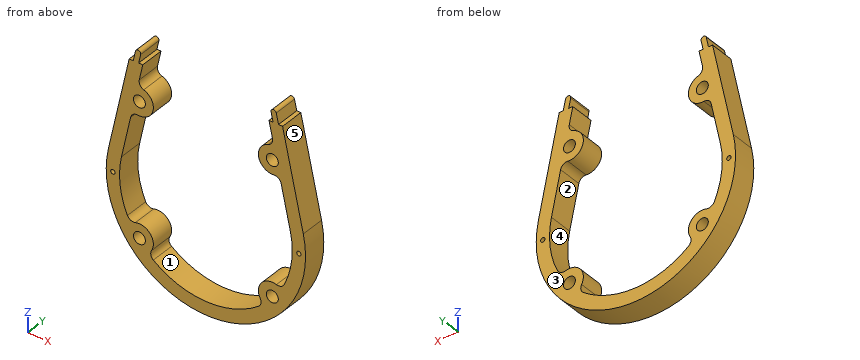
from build123d import *

# Parameters (mm, degrees)
SKETCH1_R           = 4.5
SKETCH1_R_2         = 1.65
BOSS_EXTRUDE1_DEPTH = 18


with BuildPart() as part:
    # Sketch1 → Boss-Extrude1 (new body)
    with BuildSketch(Plane(origin=(0, 0, 0), x_dir=(1, 0, 0), z_dir=(0, 1, 0))):
        with BuildLine():
            Line((-57.71713569, -88), (-54.647909803, -88))
            Line((-54.647909803, -88), (-52.972729242, -95.753217476))
            ThreePointArc((-52.972729242, -95.753217476), (-50.595460167, -97.285729058), (-49.062948585, -94.908459984))
            Line((-49.062948585, -94.908459984), (-50.555608621, -88))
            Line((-50.555608621, -88), (-47.486382735, -88))
            Line((-47.486382735, -88), (-50.121259231, -75.805033701))
            ThreePointArc((-50.121259231, -75.805033701), (-49.566331597, -72.252851185), (-46.771441988, -69.991316888))
            ThreePointArc((-46.771441988, -69.991316888), (-39.736825778, -57.782511582), (-51.184371295, -49.567010753))
            ThreePointArc((-51.184371295, -49.567010753), (-54.663630533, -48.661085559), (-56.635583446, -45.654867501))
            Line((-56.635583446, -45.654867501), (-63.533935661, -13.727309256))
            ThreePointArc((-63.533935661, -13.727309256), (-64.607519764, 7.132207931), (-59.0097537, 27.255255792))
            ThreePointArc((-59.0097537, 27.255255792), (-56.52196193, 29.718486659), (-53.028431594, 29.94621454))
            ThreePointArc((-53.028431594, 29.94621454), (-41.800877501, 33.440702001), (-40.856206486, 45.161495924))
            ThreePointArc((-40.856206486, 45.161495924), (-41.400905456, 48.61980725), (-39.543854024, 51.587630387))
            ThreePointArc((-39.543854024, 51.587630387), (0, 65), (39.543854024, 51.587630387))
            ThreePointArc((39.543854024, 51.587630387), (41.400905456, 48.61980725), (40.856206486, 45.161495924))
            ThreePointArc((40.856206486, 45.161495924), (41.800877501, 33.440702001), (53.028431594, 29.94621454))
            ThreePointArc((53.028431594, 29.94621454), (56.52196193, 29.718486659), (59.0097537, 27.255255792))
            ThreePointArc((59.0097537, 27.255255792), (64.607519764, 7.132207931), (63.533935661, -13.727309256))
            Line((63.533935661, -13.727309256), (56.635583446, -45.654867501))
            ThreePointArc((56.635583446, -45.654867501), (54.663630533, -48.661085559), (51.184371295, -49.567010753))
            ThreePointArc((51.184371295, -49.567010753), (39.736825778, -57.782511582), (46.771441988, -69.991316888))
            ThreePointArc((46.771441988, -69.991316888), (49.566331597, -72.252851185), (50.121259231, -75.805033701))
            Line((50.121259231, -75.805033701), (47.486382735, -88))
            Line((47.486382735, -88), (50.555608621, -88))
            Line((50.555608621, -88), (49.062948585, -94.908459984))
            ThreePointArc((49.062948585, -94.908459984), (50.595460167, -97.285729058), (52.972729242, -95.753217476))
            Line((52.972729242, -95.753217476), (54.647909803, -88))
            Line((54.647909803, -88), (57.71713569, -88))
            Line((57.71713569, -88), (73.308387301, -15.839202988))
            ThreePointArc((73.308387301, -15.839202988), (0, 75), (-73.308387301, -15.839202988))
            Line((-73.308387301, -15.839202988), (-57.71713569, -88))
        make_face()
        with Locations((-50, -60)):
            Circle(SKETCH1_R, mode=Mode.SUBTRACT)
        with Locations((50, -60)):
            Circle(SKETCH1_R, mode=Mode.SUBTRACT)
        with Locations((70, 0)):
            Circle(SKETCH1_R_2, mode=Mode.SUBTRACT)
        with Locations((50, 40)):
            Circle(SKETCH1_R, mode=Mode.SUBTRACT)
        with Locations((-50, 40)):
            Circle(SKETCH1_R, mode=Mode.SUBTRACT)
        with Locations((-70, 0)):
            Circle(SKETCH1_R_2, mode=Mode.SUBTRACT)
    extrude(amount=BOSS_EXTRUDE1_DEPTH)


solid = part.part
For this review, take the finished solid that the model builds, in its own axes (mm). Face numbers are marked on the shaded views. A direction names the side the tool comes from. Round coordinates to 2 decimals unless told otherwise and drop trailing zeros. Write each loop counter-clockwise with the first axis right and the second up, starting at its lowest first coordinate (ties: lowest second). Pieces come first, ordered by that corner, then holes. Notation, with made-up numbers: (-10, 10) - (-2, 10) arc R23 ccw to (-2, 25) - close; hole circle Ø1 at (66, 53). An arc over 180 degrees is marked (long way). Use a Markdown table: item, result.
Q1. Wall thickness on line 1 along X through (y, z) = (13.75, 0); line 2 along X through (y, z) = (12, -40); line 3 along X through (y, z) = (13.25, -52): over which ranges is each line inside the solid? List them lowest first.
Derived:
| item | result |
|---|---|
| line 1 | x = -75 to -71.65, -68.35 to -65, 65 to 68.35, 71.65 to 75 |
| line 2 | x = -63.44 to -54.5, -45.5 to -39.5, 39.5 to 45.5, 54.5 to 63.44 |
| line 3 | x = -54.05 to -39, 39 to 54.05 |
Q2. We need section D-D (y = 8.75). State how many separate pieces and enclosed holes the cut face has, plus the area to 3 significant figures.
Derived:
| item | result |
|---|---|
| separate pieces | 1 |
| enclosed holes | 6 |
| area | 4,700 mm2 |
Q3. We need section B-B (z = 60). Give the boundary of the cut face in (x, y).
Derived:
| item | result |
|---|---|
| outline | (-63.77, 0) - (-54.5, 0) - (-54.5, 18) - (-63.77, 18) - close; (-45.5, 0) - (-39.5, 0) - (-39.5, 18) - (-45.5, 18) - close; (39.5, 0) - (45.5, 0) - (45.5, 18) - (39.5, 18) - close; (54.5, 0) - (63.77, 0) - (63.77, 18) - (54.5, 18) - close |
Q4. We need section A-A (z = -21). Give the boundary of the cut face in (x, y), plus the area to 3 significant figures.
Derived:
| item | result |
|---|---|
| outline | (-72, 0) - (-61.51, 0) - (-61.51, 18) - (-72, 18) - close; (61.51, 0) - (72, 0) - (72, 18) - (61.51, 18) - close |
| area | 377 mm2 |
Q5. Clearance check with flat-ended pins moving along their axes: pin 1 (1.5 mm diameter, centred on y = 12, z = -39, fed in from -X); pin 2 (1.5 mm diameter, centred on x = -48.5, y = 9, fed in from +Z); pin 3 (3.5 mm diameter, centred on x = -56.5, y = 11, fed in from +Z). State where each tip first meets the part, or that it passes through.
Derived:
| item | result |
|---|---|
| pin 1 | stops at x = -64.51 |
| pin 2 | stops at z = 96.27 |
| pin 3 | stops at z = 88 |
Q6. We need section C-C (x = 0). Give the boundary of the cut face in (y, z), plus the area to 3 significant figures.
Derived:
| item | result |
|---|---|
| outline | (0, -75) - (18, -75) - (18, -65) - (0, -65) - close |
| area | 180 mm2 |
Q7. Machinability: for the marked faces 4 and 5, which of the approach directions +Z, -Z, +X, -X, +Y, -Y give a long, thin tool a straight path to every point of the face, cutting with its end or side? Answer none if there is none.
Derived:
| item | result |
|---|---|
| face 4 | +Y, -Y |
| face 5 | +Z, +X, +Y, -Y |
Q8. The part is to be moulded in two halves that separate along Z. For the marked faces 1, 2 and 3, say which applies: pulls with the +Z half, pulls with the -Z half, needs draft (parallel to the pull), parting line crosses it, or undercut.
Derived:
| item | result |
|---|---|
| face 1 | pulls with the +Z half |
| face 2 | undercut |
| face 3 | needs draft |
